Solid Edge part; units mm, degrees
sketch "Sketch1" plane through (0, 0, 0) normal (0, 0, 1) x (1, 0, 0)
  circle A0 centre (0, 0) radius 7
extrude "Protrusion1" add sketch "Sketch1" along normal blind 6
sketch "Sketch2" plane through (0, 0, 0) normal (0, -1, 0) x (1, 0, 0)
  line L0 (-4.75, 6) -> (-7, 0)
revolve "RevolvedCutout1" cut sketch "Sketch2" angle 360 about axis through (0, 0, 54) along (0, 0, -1) material side at (-5.9218, 0, 3.0176)
hole "Hole_1" at (0, 0, 6) direction (0, 0, -1) diameter 6.647 end through all
sketch "Sketch3" plane through (0, 0, 0) normal (1, 0, 0) x (0, 1, 0)
  line L0 (-15.3653, 14.4486) -> (-13.7058, 4.9657)
  arc A0 (-13.7058, 4.9657) -> (-7.7956, 0) centre (-7.7956, 6) ccw
  line L1 (-7.7956, 0) -> (-6.0543, 0)
  line L2 (-3.75, 6) -> (-6.0543, 0)
  line L3 (-4.75, 6) -> (-3.75, 6)
  line L4 (-6.5, 16) -> (-4.75, 6)
  line L5 (-6.5, 16) -> (-15.3653, 14.4486)
extrude "ExtrudedProtrusion_3" add sketch "Sketch3" along normal mid plane 5
mirror "Mirror1" about plane through (0, 0, 0) normal (0, -1, 0) of "ExtrudedProtrusion_3"
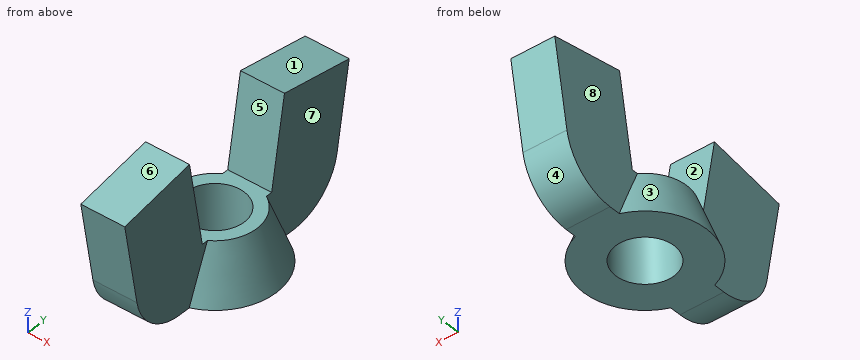
Can you work these out from the model? Positions are in its coordinate system, mm. Face numbers are marked on the shaded views. A direction names the side the tool comes from. Give positions to 0.01 mm unless a question says otherwise; leave off trailing zeros. Loops run counter-clockwise (first coordinate to the right, second up) from the corner with the lowest first, then second, coordinate; pieces in that order, holes last. Notation, with made-up numbers: (84, 16.25) -> (112, 16.25) arc R22 ccw to (112, 37.25) -> close; hole circle Ø2 at (-22, 44). An arc over 180 degrees is marked (long way). Write item = value, one per line.
1) Suppose I cut it at C-C on z = 13. Write out the boundary of the cut face in (x, y) (3 decimals).
Check result:
outline = (-2.5, -15.112) -> (2.5, -15.112) -> (2.5, -5.975) -> (-2.5, -5.975) -> close; (-2.5, 5.975) -> (2.5, 5.975) -> (2.5, 15.112) -> (-2.5, 15.112) -> close
2) Will these pins go through, and if not, where does the flat tip stop? pin 1 (1 mm diameter, centred on y = 6, z = 3, fed in from -X); pin 2 (3 mm diameter, centred on x = 2, y = 0, fed in from +Z); pin 3 (1 mm diameter, centred on x = -0.5, z = 9.5, fed in from -Y).
Check result:
pin_1 = -2.5
pin_2 = 6
pin_3 = -14.59
3) Suppose I cut it at A-A on x = 0. Write out the boundary of the cut face in (y, z), then the cut area to 3 significant figures.
Check result:
outline = (-15.37, 14.45) -> (-13.71, 4.97) arc R6 ccw to (-7.8, 0) -> (-3.32, 0) -> (-3.32, 6) -> (-4.75, 6) -> (-6.5, 16) -> close; (3.32, 0) -> (7.8, 0) arc R6 ccw to (13.71, 4.97) -> (15.37, 14.45) -> (6.5, 16) -> (4.75, 6) -> (3.32, 6) -> close
area = 279 mm2
4) Suppose I cut it at B-B on y = 0. Write out the boundary of the cut face in (x, z).
Check result:
outline = (-7, 0) -> (-3.32, 0) -> (-3.32, 6) -> (-4.75, 6) -> close; (3.32, 0) -> (7, 0) -> (4.75, 6) -> (3.32, 6) -> close
5) I need wall thicknesses on L1, parallel to X at y = 7, z = 6.5; L2, parallel to Y at x = 0, z = 4.7; L3, parallel to Y at x = -1.75, z = 3.5. Which ranges of each line are inside material? Lowest first, please. Write a range as from..to.
Check result:
L1 = -2.5..2.5
L2 = -13.65..-3.32, 3.32..13.65
L3 = -13.25..-2.83, 2.83..13.25
6) Suppose I cut it at D-D on x = -1.5. Write out the boundary of the cut face in (y, z), then the cut area to 3 significant figures.
Check result:
outline = (-15.37, 14.45) -> (-13.71, 4.97) arc R6 ccw to (-7.8, 0) -> (-2.97, 0) -> (-2.97, 6) -> (-4.75, 6) -> (-6.5, 16) -> close; (2.97, 0) -> (7.8, 0) arc R6 ccw to (13.71, 4.97) -> (15.37, 14.45) -> (6.5, 16) -> (4.75, 6) -> (2.97, 6) -> close
area = 283 mm2
7) Thinking about a two-plate mould opening in Y: for the marked faces 1, 2 and 3, which applies, released by +Y, released by -Y, zero draft, split by the parting line, or undercut?
Check result:
face_1 = released by +Y
face_2 = undercut
face_3 = split by the parting line
8) For the marked faces 4, 5, 6, 7 and 8, which set-ups out of +Z, -Z, +X, -X, +Y, -Y let a thin tool reach every point of the face, with its end or its side?
Check result:
face_4 = -Z, +X, -X, +Y
face_5 = +Z, +X, -X
face_6 = +Z, +X, -X, -Y
face_7 = +Z, +X, +Y
face_8 = +Z, -X, +Y
